Autodesk Inventor part; units mm, degrees
ref_plane "Plan YZ" through (0, 0, 0) normal (1, 0, 0) x (0, 1, 0)
ref_plane "Plan XZ" through (0, 0, 0) normal (0, 1, 0) x (-1, 0, 0)
ref_plane "Plan XY" through (0, 0, 0) normal (0, 0, 1) x (1, 0, 0)
sketch "Esquisse7" plane through (0, 0, 0) normal (0, 0, 1) x (1, 0, 0)
  line L0 (-40.2, -26) -> (-40.2, 26)
  line L1 (-40.2, 26) -> (-35.2, 26)
  line L2 (-35.2, 26) -> (-35.2, 29)
  line L3 (-35.2, 29) -> (-20.2, 29)
  line L4 (-20.2, 29) -> (-20.2, 26)
  line L5 (20.2, 26) -> (20.2, 29)
  line L6 (20.2, 29) -> (35.2, 29)
  line L7 (35.2, 29) -> (35.2, 26)
  line L8 (35.2, 26) -> (40.2, 26)
  line L9 (40.2, 26) -> (40.2, -26)
  line L10 (40.2, -26) -> (35.2, -26)
  line L11 (35.2, -26) -> (35.2, -29)
  line L12 (35.2, -29) -> (20.2, -29)
  line L13 (20.2, -29) -> (20.2, -26)
  line L14 (-20.2, -26) -> (-20.2, -29)
  line L15 (-35.2, -29) -> (-35.2, -26)
  line L16 (-40.2, -26) -> (-35.2, -26)
  line L17 (-35.2, -29) -> (-20.2, -29)
  line L18 (0, -40.6) -> (0, 40.6) construction
  line L19 (-56.28, 0) -> (56.28, 0) construction
  line L20 (-20.2, -26) -> (-7.5, -26)
  line L21 (7.5, -26) -> (20.2, -26)
  line L22 (-20.2, 26) -> (-7.5, 26)
  line L23 (7.5, 26) -> (20.2, 26)
  line L24 (-7.5, -26) -> (7.5, -26)
  line L25 (-7.5, 26) -> (7.5, 26)
  point P0 (0, 0)
  dimension "d33" = 52
  dimension "d34" = 5
  dimension "d35" = 3
  dimension "d36" = 15
  dimension "d51" = 80.4
extrude "Extrusion3" add sketch "Esquisse7" along normal blind 3
chamfer "Chanfrein5" distance 1 angle 45 8 edges at (-20.2, 29, 1.5) (-35.2, 29, 1.5) (20.2, 29, 1.5) (35.2, 29, 1.5) (35.2, -29, 1.5) (20.2, -29, 1.5) (-20.2, -29, 1.5) (-35.2, -29, 1.5)
sketch "Esquisse10" plane through (0, 0, 3) normal (0, 0, 1) x (1, 0, 0)
  line L0 (-34.2, -29) -> (-35.2, -28) construction
  line L1 (-34.2, -29) -> (-21.2, -29) construction
  line L2 (-20.2, -28) -> (-21.2, -29) construction
  line L3 (-20.2, -28) -> (-20.2, -26) construction
  line L4 (-20.2, -26) -> (20.2, -26) construction
  line L5 (20.2, -26) -> (20.2, -28) construction
  line L6 (21.2, -29) -> (20.2, -28) construction
  line L7 (21.2, -29) -> (34.2, -29) construction
  line L8 (35.2, -28) -> (34.2, -29) construction
  line L9 (35.2, -28) -> (35.2, -26) construction
  line L10 (35.2, -26) -> (40.2, -26) construction
  line L11 (40.2, -26) -> (40.2, 26) construction
  line L12 (40.2, 26) -> (35.2, 26) construction
  line L13 (35.2, 26) -> (35.2, 28) construction
  line L14 (34.2, 29) -> (35.2, 28) construction
  line L15 (34.2, 29) -> (21.2, 29) construction
  line L16 (20.2, 28) -> (21.2, 29) construction
  line L17 (20.2, 28) -> (20.2, 26) construction
  line L18 (20.2, 26) -> (-20.2, 26) construction
  line L19 (-20.2, 26) -> (-20.2, 28) construction
  line L20 (-21.2, 29) -> (-20.2, 28) construction
  line L21 (-21.2, 29) -> (-34.2, 29) construction
  line L22 (-35.2, 28) -> (-34.2, 29) construction
  line L23 (-35.2, 28) -> (-35.2, 26) construction
  line L24 (-35.2, 26) -> (-40.2, 26) construction
  line L25 (-40.2, 26) -> (-40.2, -26) construction
  line L26 (-40.2, -26) -> (-35.2, -26) construction
  line L27 (-35.2, -26) -> (-35.2, -28) construction
  point P0 (0, 0)
hole "Perçage4" at (-35.2, 26, 3) at (-20.2, 26, 3) at (20.2, 26, 3) at (35.2, 26, 3) at (-35.2, -26, 3) at (-20.2, -26, 3) at (20.2, -26, 3) at (35.2, -26, 3) direction (0, 0, -1) diameter 1 end through all
properties part number "P1704_204" material "Plastique PMMA"
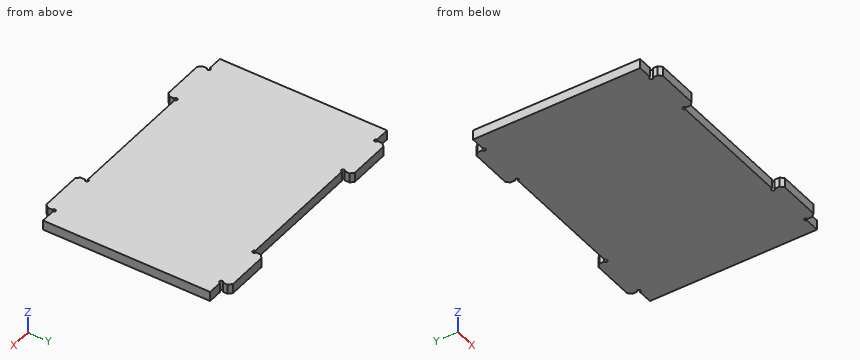
Read the model definition and answer for the solid it produces. Units are mm, in the model's axes. Round coordinates to 2 decimals unless told otherwise and drop trailing zeros. Loops run counter-clockwise (first coordinate to the right, second up) from the corner with the lowest first, then second, coordinate; pieces in that order, holes last.
Q1. Each of these flat-tipped pins is pushed along its axis until it touches: pin 1 (0.9 mm diameter, centred on x = 37, z = 1, fed in from -Y); pin 2 (1.2 mm diameter, centred on y = 27, z = 1.5, fed in from +X); pin 3 (0.9 mm diameter, centred on x = -37.5, z = 1.5, fed in from +Y); pin 4 (8 mm diameter, centred on x = 21, y = 13, fed in from -Z). Where does it stop, or does it pass through?
Q2. Consider probe 1 along Y at (x, z) = (35, 1.7); probe 2 along Y at (x, z) = (-11, 1). Determine where each line is inside the solid, lowest interval first.
Q3. Section A-A on x = -14 is taken. Write down the section's boundary in (y, z), and give its area (3 significant figures).
Output:
1. pin 1: stops at y = -26
1. pin 2: stops at x = 35.2
1. pin 3: stops at y = 26
1. pin 4: stops at z = 0
2. probe 1: y = -28.2 to -26.46, -25.54 to 25.54, 26.46 to 28.2
2. probe 2: y = -26 to 26
3. outline: (-26, 0) - (26, 0) - (26, 3) - (-26, 3) - close
3. area: 156 mm2
